Verification items for this drawing (mm, ordinates from the low corner). A direction names the side the tool comes from. Coordinates: 2 decimals unless noted, no trailing zeros. Loops run counter-clockwise (first coordinate to the right, second up) from the corner with the lowest first, then second, coordinate; pieces in that order, holes last. Notation, with made-up numbers: (57.5, 88.5) -> (67.5, 88.5) arc R16 ccw to (67.5, 108.5) -> close; hole circle Ø10 at (63.5, 31). An arc over 180 degrees is marked (long way). Write item = value, one per line.
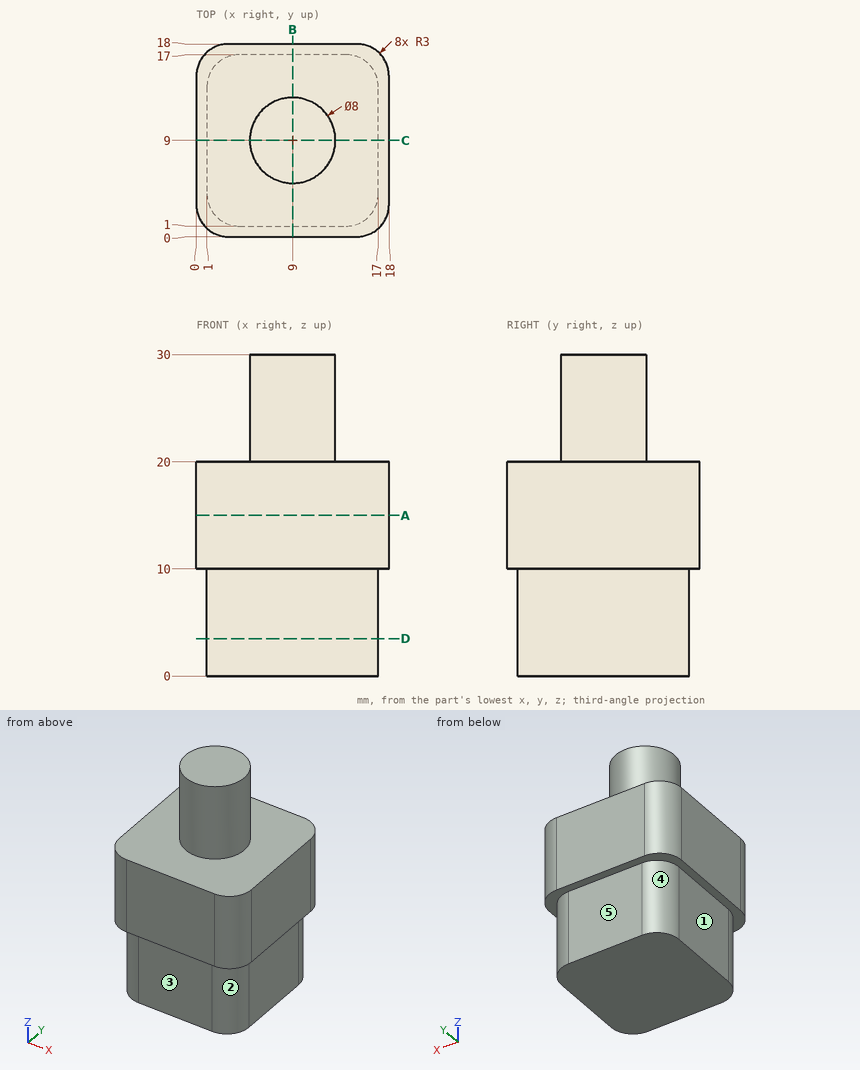
1) Sectioned sample at B-B, the plane x = 9. Record the cut outline in (y, z).
Ans:
outline = (0, 10) -> (1, 10) -> (1, 0) -> (17, 0) -> (17, 10) -> (18, 10) -> (18, 20) -> (13, 20) -> (13, 30) -> (5, 30) -> (5, 20) -> (0, 20) -> close
2) Sectioned sample at A-A, the plane z = 15. Record the cut outline in (x, y).
Ans:
outline = (0, 3) arc R3 ccw to (3, 0) -> (15, 0) arc R3 ccw to (18, 3) -> (18, 15) arc R3 ccw to (15, 18) -> (3, 18) arc R3 ccw to (0, 15) -> close
3) Depth check by flat-ended pin: pin 1 Ø3 at (x, z) = (7, 4.5) entering from +Y; pin 2 Ø3 at (y, z) = (11.5, 5.5) entering from -X; pin 3 Ø3 at (x, z) = (9, 4.5) entering from -Y; pin 4 Ø3 at (y, z) = (15.5, 22) entering from +X. Enter the tip coordinate at first touch or a pass-through.
Ans:
pin_1 = 17
pin_2 = 1
pin_3 = 1
pin_4 = through
4) Material ranges on line 1 (X direction, y = 11, z = 7); line 2 (Z direction, x = 6.25, y = 5.5); line 3 (Z direction, x = 9.25, y = 17.25), recorded low to high.
Ans:
line_1 = 1 to 17
line_2 = 0 to 20
line_3 = 10 to 20
5) Sectioned sample at D-D, the plane z = 3.5. Record the cut outline in (x, y), plus the area to 3 significant figures.
Ans:
outline = (1, 4) arc R3 ccw to (4, 1) -> (14, 1) arc R3 ccw to (17, 4) -> (17, 14) arc R3 ccw to (14, 17) -> (4, 17) arc R3 ccw to (1, 14) -> close
area = 248 mm2
6) Tool access check on the marked faces 1, 2, 3, 4 and 5. Record the directions out of +Z, -Z, +X, -X, +Y, -Y that give a thin tool (end or side, any length) a straight path to the whole face; none if there is none.
Ans:
face_1 = -Z, -X, +Y, -Y
face_2 = -Z, +X, -Y
face_3 = -Z, +X, -X, -Y
face_4 = -Z, -X, +Y
face_5 = -Z, +X, -X, +Y
